```python
from build123d import *

# Parameters (mm, degrees)
SKETCH1_W           = 365
SKETCH1_H           = 370
BOSS_EXTRUDE1_DEPTH = 3
SKETCH2_W           = 365
SKETCH2_H           = 135
CUT_EXTRUDE1_DEPTH  = 10
SKETCH3_R           = 1.25
SKETCH3_R_2         = 8
CUT_EXTRUDE2_DEPTH  = 10
SKETCH4_R           = 5.3
SKETCH4_R_2         = 1.2
CUT_EXTRUDE3_DEPTH  = 10
SKETCH5_W           = 258
SKETCH5_H           = 82.769773142
CUT_EXTRUDE4_DEPTH  = 10
SKETCH6_W           = 15
SKETCH6_H           = 40
CUT_EXTRUDE5_DEPTH  = 10
CUT_EXTRUDE6_DEPTH  = 10
CUT_EXTRUDE7_DEPTH  = 10
SKETCH9_R           = 2.2
CUT_EXTRUDE8_DEPTH  = 10
FILLET1_R           = 10
CUT_EXTRUDE9_DEPTH  = 10
SKETCH11_R          = 2.2
CUT_EXTRUDE10_DEPTH = 10
SKETCH12_W          = 38.5
SKETCH12_H          = 60
BOSS_EXTRUDE2_DEPTH = 3
LPATTERN1_COUNT     = 2
LPATTERN1_PITCH     = 230
FILLET2_R           = 5


with BuildPart() as part:
    # Sketch1 → Boss-Extrude1 (new body)
    with BuildSketch(Plane(origin=(0, 0, 0), x_dir=(1, 0, 0), z_dir=(0, 1, 0))):
        Rectangle(SKETCH1_W, SKETCH1_H)
    extrude(amount=BOSS_EXTRUDE1_DEPTH)

    # Sketch2 → Cut-Extrude1 (cut)
    with BuildSketch(Plane(origin=(0, 3, 0), x_dir=(1, 0, 0), z_dir=(0, 1, 0))):
        with Locations((0, -117.5)):
            Rectangle(SKETCH2_W, SKETCH2_H)
    extrude(amount=-CUT_EXTRUDE1_DEPTH, mode=Mode.SUBTRACT)

    # Sketch3 → Cut-Extrude2 (cut)
    with BuildSketch(Plane(origin=(0, 3, 0), x_dir=(1, 0, 0), z_dir=(0, 1, 0))):
        with Locations((-173.485281374, 155.985281374)):
            Circle(SKETCH3_R)
        with Locations((-173.485281374, 139.014718626)):
            Circle(SKETCH3_R)
        with Locations((-156.514718626, 155.985281374)):
            Circle(SKETCH3_R)
        with Locations((-156.514718626, 139.014718626)):
            Circle(SKETCH3_R)
        with Locations((-165, 147.5)):
            Circle(SKETCH3_R_2)
        with Locations((156.514718626, 155.985281374)):
            Circle(SKETCH3_R)
        with Locations((173.485281374, 155.985281374)):
            Circle(SKETCH3_R)
        with Locations((173.485281374, 139.014718626)):
            Circle(SKETCH3_R)
        with Locations((156.514718626, 139.014718626)):
            Circle(SKETCH3_R)
        with Locations((165, 147.5)):
            Circle(SKETCH3_R_2)
    cut_extrude2 = extrude(amount=-CUT_EXTRUDE2_DEPTH, mode=Mode.SUBTRACT)

    # Sketch4 → Cut-Extrude3 (cut)
    with BuildSketch(Plane(origin=(0, 3, 0), x_dir=(1, 0, 0), z_dir=(0, 1, 0))):
        with Locations((-169, -17.5)):
            Circle(SKETCH4_R)
        with Locations((-169, -9.5)):
            Circle(SKETCH4_R_2)
        with Locations((-169, -25.5)):
            Circle(SKETCH4_R_2)
        with Locations((-161, -17.674075017)):
            Circle(SKETCH4_R_2)
        with Locations((-177, -17.674075017)):
            Circle(SKETCH4_R_2)
    cut_extrude3 = extrude(amount=-CUT_EXTRUDE3_DEPTH, mode=Mode.SUBTRACT)

    # Mirror1: Cut-Extrude3 across plane
    add(cut_extrude3.mirror(Plane(origin=(0, 0, 0), x_dir=(0, 0, 1), z_dir=(1, 0, 0))), mode=Mode.SUBTRACT)

    # Sketch5 → Cut-Extrude4 (cut)
    with BuildSketch(Plane(origin=(0, 3, 0), x_dir=(1, 0, 0), z_dir=(0, 1, 0))):
        with Locations((0, -8.615113429)):
            Rectangle(SKETCH5_W, SKETCH5_H)
    extrude(amount=-CUT_EXTRUDE4_DEPTH, mode=Mode.SUBTRACT)

    # Sketch6 → Cut-Extrude5 (cut)
    with BuildSketch(Plane(origin=(0, 3, 0), x_dir=(1, 0, 0), z_dir=(0, 1, 0))):
        with Locations((-136.5, -30)):
            Rectangle(SKETCH6_W, SKETCH6_H)
    cut_extrude5 = extrude(amount=-CUT_EXTRUDE5_DEPTH, mode=Mode.SUBTRACT)

    # Mirror2: Cut-Extrude5 across plane
    add(cut_extrude5.mirror(Plane(origin=(0, 0, 0), x_dir=(0, 0, 1), z_dir=(1, 0, 0))), mode=Mode.SUBTRACT)

    # Sketch7 → Cut-Extrude6 (cut)
    with BuildSketch(Plane(origin=(0, 3, 0), x_dir=(1, 0, 0), z_dir=(0, 1, 0))):
        with BuildLine():
            ThreePointArc((-24.767233991, 32.769773142), (-32.340788408, 44.118168841), (-35, 57.5))
            Line((-35, 57.5), (-35, 32.769773142))
            Line((-35, 32.769773142), (-24.767233991, 32.769773142))
        make_face()
        with BuildLine():
            ThreePointArc((34.808648008, 61.154863037), (-1.829934385, 92.452129265), (-35, 57.5))
            ThreePointArc((-35, 57.5), (-32.340788408, 44.118168841), (-24.767233991, 32.769773142))
            Line((-24.767233991, 32.769773142), (24.767233991, 32.769773142))
            ThreePointArc((24.767233991, 32.769773142), (31.697667218, 42.658912002), (34.854759109, 54.31475787))
            Line((34.854759109, 54.31475787), (34.808648008, 61.154863037))
        make_face()
        with BuildLine():
            Line((35, 32.769773142), (34.854759109, 54.31475787))
            ThreePointArc((34.854759109, 54.31475787), (31.697667218, 42.658912002), (24.767233991, 32.769773142))
            Line((24.767233991, 32.769773142), (35, 32.769773142))
        make_face()
    extrude(amount=-CUT_EXTRUDE6_DEPTH, mode=Mode.SUBTRACT)

    # Sketch8 → Cut-Extrude7 (cut)
    with BuildSketch(Plane(origin=(0, 3, 0), x_dir=(1, 0, 0), z_dir=(0, 1, 0))):
        with BuildLine():
            Line((-169.5, 52), (-139.5, 52))
            ThreePointArc((-139.5, 52), (-135.964466094, 53.464466094), (-134.5, 57))
            Line((-134.5, 57), (-134.5, 77))
            ThreePointArc((-134.5, 77), (-135.964466094, 80.535533906), (-139.5, 82))
            Line((-139.5, 82), (-169.5, 82))
            ThreePointArc((-169.5, 82), (-173.035533906, 80.535533906), (-174.5, 77))
            Line((-174.5, 77), (-174.5, 57))
            ThreePointArc((-174.5, 57), (-173.035533906, 53.464466094), (-169.5, 52))
        make_face()
    cut_extrude7 = extrude(amount=-CUT_EXTRUDE7_DEPTH, mode=Mode.SUBTRACT)

    # Mirror3: Cut-Extrude7 across plane
    add(cut_extrude7.mirror(Plane(origin=(0, 0, 0), x_dir=(0, 0, 1), z_dir=(1, 0, 0))), mode=Mode.SUBTRACT)

    # Sketch9 → Cut-Extrude8 (cut)
    with BuildSketch(Plane(origin=(0, 3, 0), x_dir=(1, 0, 0), z_dir=(0, 1, 0))):
        with Locations((-136.5, -2)):
            Circle(SKETCH9_R)
        with Locations((-136.5, 43)):
            Circle(SKETCH9_R)
        with Locations((-136.5, 88)):
            Circle(SKETCH9_R)
        with Locations((-136.5, 133)):
            Circle(SKETCH9_R)
        with Locations((-136.5, 178)):
            Circle(SKETCH9_R)
        with Locations((136.5, 178)):
            Circle(SKETCH9_R)
        with Locations((136.5, 133)):
            Circle(SKETCH9_R)
        with Locations((136.5, 88)):
            Circle(SKETCH9_R)
        with Locations((136.5, 43)):
            Circle(SKETCH9_R)
        with Locations((136.5, -2)):
            Circle(SKETCH9_R)
    extrude(amount=-CUT_EXTRUDE8_DEPTH, mode=Mode.SUBTRACT)

    # Fillet1
    fillet1_edges = [part.edges().sort_by_distance(p)[0] for p in [
        (-129, 1.5, -32.769773142),
        (129, 1.5, -32.769773142),
    ]]
    fillet(fillet1_edges, radius=FILLET1_R)

    # Sketch10 → Cut-Extrude9 (cut)
    with BuildSketch(Plane(origin=(0, 3, 0), x_dir=(1, 0, 0), z_dir=(0, 1, 0))):
        with BuildLine():
            Line((102.5, 72.769773142), (62.5, 72.769773142))
            ThreePointArc((62.5, 72.769773142), (58.964466094, 74.234239236), (57.5, 77.769773142))
            Line((57.5, 77.769773142), (57.5, 147.769773142))
            ThreePointArc((57.5, 147.769773142), (58.964466094, 151.305307048), (62.5, 152.769773142))
            Line((62.5, 152.769773142), (102.5, 152.769773142))
            ThreePointArc((102.5, 152.769773142), (106.035533906, 151.305307048), (107.5, 147.769773142))
            Line((107.5, 147.769773142), (107.5, 77.769773142))
            ThreePointArc((107.5, 77.769773142), (106.035533906, 74.234239236), (102.5, 72.769773142))
        make_face()
        with BuildLine():
            Line((-57.5, 77.769773142), (-57.5, 147.769773142))
            ThreePointArc((-57.5, 147.769773142), (-58.964466094, 151.305307048), (-62.5, 152.769773142))
            Line((-62.5, 152.769773142), (-102.5, 152.769773142))
            ThreePointArc((-102.5, 152.769773142), (-106.035533906, 151.305307048), (-107.5, 147.769773142))
            Line((-107.5, 147.769773142), (-107.5, 77.769773142))
            ThreePointArc((-107.5, 77.769773142), (-106.035533906, 74.234239236), (-102.5, 72.769773142))
            Line((-102.5, 72.769773142), (-62.5, 72.769773142))
            ThreePointArc((-62.5, 72.769773142), (-58.964466094, 74.234239236), (-57.5, 77.769773142))
        make_face()
    extrude(amount=-CUT_EXTRUDE9_DEPTH, mode=Mode.SUBTRACT)

    # Sketch11 → Cut-Extrude10 (cut)
    with BuildSketch(Plane(origin=(0, 3, 0), x_dir=(1, 0, 0), z_dir=(0, 1, 0))):
        with Locations((20, 145)):
            Circle(SKETCH11_R)
        with Locations((20, 105)):
            Circle(SKETCH11_R)
        with Locations((-20, 105)):
            Circle(SKETCH11_R)
        with Locations((-20, 145)):
            Circle(SKETCH11_R)
    extrude(amount=-CUT_EXTRUDE10_DEPTH, mode=Mode.SUBTRACT)

    # Sketch12 → Boss-Extrude2 (add)
    with BuildSketch(Plane(origin=(0, 3, 0), x_dir=(1, 0, 0), z_dir=(0, 1, 0))):
        with Locations((-163.25, -80)):
            Rectangle(SKETCH12_W, SKETCH12_H)
    boss_extrude2 = extrude(amount=-BOSS_EXTRUDE2_DEPTH)

    # Mirror4: Boss-Extrude2 across plane
    add(boss_extrude2.mirror(Plane(origin=(0, 0, 0), x_dir=(0, 0, 1), z_dir=(1, 0, 0))))

    # LPattern1: Cut-Extrude2 ×2
    with Locations(*[(0, 0, i * LPATTERN1_PITCH) for i in range(1, LPATTERN1_COUNT)]):
        add(cut_extrude2, mode=Mode.SUBTRACT)

    # Fillet2
    fillet2_edges = [part.edges().sort_by_distance(p)[0] for p in [
        (35, 1.5, -32.769773142),
        (-35, 1.5, -32.769773142),
        (-182.5, 1.5, 110),
        (-144, 1.5, 110),
        (182.5, 1.5, 110),
        (144, 1.5, 110),
        (-182.5, 1.5, -185),
        (182.5, 1.5, -185),
    ]]
    fillet(fillet2_edges, radius=FILLET2_R)


solid = part.part
```
Build history of the part. All positions in model axes, mm. A direction names the side the tool comes from. Give positions to 0.01 mm unless a question says otherwise; leave off trailing zeros. Loops run counter-clockwise (first coordinate to the right, second up) from the corner with the lowest first, then second, coordinate; pieces in that order, holes last.
1) Two-plate mould, pull along X, no slides. Class faces 3 (the face through (3, 0, -105)), 4 (the face through (163.27, 1.52, -139.69)): released by +X, released by -X, zero draft, split by the parting line, or undercut.
Values follow:
face 3: zero draft
face 4: undercut
2) Band-saw the part on C-C on y = 0.7. State how many separate pieces and enclosed holes the cut face has, then the cut area to 3 significant figures.
Values follow:
separate pieces: 1
enclosed holes: 48
area: 52,600 mm2
3) Band-saw the part on B-B on x = 71.5. List the corners of the cut face in (y, z).
Values follow:
outline: (0, -185) - (3, -185) - (3, -152.77) - (0, -152.77) - close; (0, -72.77) - (3, -72.77) - (3, -32.77) - (0, -32.77) - close
4) 3-axis set-ups, long thin cutter, end or side, ignore diameter. For faces 1 (the face through (-166.041, 1.521, 74.568)), 2 (the face through (126.15, 1.48, -29.76)): which of +Z, -Z, +X, -X, +Y, -Y reach the whole face in a straight line?
Values follow:
face 1: +Y, -Y
face 2: +Z, +Y, -Y
5) Probe line 1 along X through (y, z) = (2.4, -100); line 2 along X through (y, z) = (1.4, 2); line 3 along X through (y, z) = (2.2, -43). List the from-to ranges inside material, lowest first.
Values follow:
line 1: x = -182.5 to -107.5, -57.5 to 57.5, 107.5 to 182.5
line 2: x = -182.5 to -138.7, -134.3 to -129, 129 to 134.3, 138.7 to 182.5
line 3: x = -182.5 to -138.7, -134.3 to -35, 34.93 to 134.3, 138.7 to 182.5
6) Drop flat-ended pins along their axis: P1, Ø7, axis at x = -136.5, z = -43, coming from the -Y side; P2, Ø1.5, axis at x = 23, y = 0.5, coming from the +Z side. Give the stop position or say it passes through.
Values follow:
P1: stops at y = 0
P2: stops at z = -83.21
7) Band-saw the part on A-A on z = 57. List the corners of the cut face in (x, y), then the cut area to 3 significant figures.
Values follow:
outline: (-182.5, 0) - (-144, 0) - (-144, 3) - (-182.5, 3) - close; (144, 0) - (182.5, 0) - (182.5, 3) - (144, 3) - close
area: 231 mm2
